```python
from build123d import *

# Parameters (mm, degrees)
ESQUISSE1_R                  = 2.5
BOSS_EXTRU_1_DEPTH           = 25
ESQUISSE2_R                  = 4.5
BOSS_EXTRU_2_DEPTH           = 1.5
ENL_V_MAT_EXTRU_1_DEPTH      = 28.25344015
ENL_V_MAT_EXTRU_1_DEPTH_BACK = 10
ESQUISSE3_R                  = 2


with BuildPart() as part:
    # Esquisse1 → Boss.-Extru.1 (new body)
    with BuildSketch(Plane.XY):
        Circle(ESQUISSE1_R)
    extrude(amount=BOSS_EXTRU_1_DEPTH)

    # Esquisse2 → Boss.-Extru.2 (add)
    with BuildSketch(Plane.XY):
        Circle(ESQUISSE2_R)
        Polygon((-1.718731116, -0.115769453), (-1.718731116, 0.115769453), (-0.115769453, 0.115769453), (-0.115769453, 1.718731116), (0.115769453, 1.718731116), (0.115769453, 0.115769453), (1.718731116, 0.115769453), (1.718731116, -0.115769453), (0.115769453, -0.115769453), (0.115769453, -1.718731116), (-0.115769453, -1.718731116), (-0.115769453, -0.115769453), align=None, mode=Mode.SUBTRACT)
    extrude(amount=-BOSS_EXTRU_2_DEPTH)

    # Esquisse3 → Enlèv. mat.-Extru.1 (cut, two sides: drawn at the far end of the back side and taken through both)
    with BuildSketch(Plane.XY.offset(25).offset(-ENL_V_MAT_EXTRU_1_DEPTH_BACK)):
        with Locations(Location((0, 0, 0), (0, 0, 180))):
            Circle(ESQUISSE3_R)
    extrude(amount=ENL_V_MAT_EXTRU_1_DEPTH + ENL_V_MAT_EXTRU_1_DEPTH_BACK, mode=Mode.SUBTRACT)


solid = part.part
```
Geometry check sheet. Reference: the model listing, model coordinates, mm. A direction names the side the tool comes from. Give positions to 0.01 mm unless a question says otherwise; leave off trailing zeros. Write each loop counter-clockwise with the first axis right and the second up, starting at its lowest first coordinate (ties: lowest second). Pieces come first, ordered by that corner, then holes.
1) Release check for a two-part mould opening along X. For faces 4 (the flat face through (-1, 0.116, -1)), 5 (the flat face through (-1, 2, 25)), 6 (the cylindrical face through (-0.59, 4.46, -0.74)), 7 (the flat face through (-1, -0.116, -1)) record: pulls with the +X half, pulls with the -X half, needs draft (parallel to the pull), parting line crosses it, or undercut.
2) Section check A-A, the plane y = 1. Record the boundary of the cut face in (x, z).
3) Access from +Z, -Z, +X, -X, +Y, -Y to the whole of each face (thin tool, end or side, straight path). Record for faces 1 (the cylindrical face through (0, 2, 20)), 2 (the flat face through (1, -1, -1.5)), 3 (the flat face through (-0.116, -1, -1)).
4) Material ranges on L1, parallel to Y at x = 0, z = 23; L2, parallel to Z at x = 0.75, y = -1.75; L3, parallel to Z at x = 3.25, y = -0.25, recorded low to high.
5) Section check C-C, the plane z = 21. Record the boundary of the cut face in (x, y), and give its area (3 significant figures).
6) Gauge pin test, flat ends, axial feed: pin 1 (1 mm diameter, centred on y = -1, z = 16.5, fed in from -X); pin 2 (1 mm diameter, centred on x = 1.5, z = 5.5, fed in from -Y); pin 3 (1 mm diameter, centred on x = 1, z = 16.5, fed in from +Y). Record the tip position at first contact, or that the pin passes through.
7) Section check B-B, the plane z = 9.25. Record the boundary of the cut face in (x, y).
Computed:
1. face 4: undercut
1. face 5: needs draft
1. face 6: parting line crosses it
1. face 7: undercut
2. outline: (-4.39, -1.5) - (-0.12, -1.5) - (-0.12, 0) - (0.12, 0) - (0.12, -1.5) - (4.39, -1.5) - (4.39, 0) - (2.29, 0) - (2.29, 25) - (1.73, 25) - (1.73, 15) - (-1.73, 15) - (-1.73, 25) - (-2.29, 25) - (-2.29, 0) - (-4.39, 0) - close
3. face 1: +Z
3. face 2: -Z, +X, -X, +Y, -Y
3. face 3: -Z
4. L1: y = -2.5 to -2, 2 to 2.5
4. L2: z = -1.5 to 15
4. L3: z = -1.5 to 0
5. outline: circle Ø5 at (0, 0); hole circle Ø4 at (0, 0)
5. area: 7.07 mm2
6. pin 1: stops at x = -2.45
6. pin 2: stops at y = -2.29
6. pin 3: stops at y = 2.45
7. outline: circle Ø5 at (0, 0)
